```python
from build123d import *

# Parameters (mm, degrees)
BOSS_EXTRUDE1_DEPTH = 15
SKETCH6_R           = 15
SKETCH6_R_2         = 3
BOSS_EXTRUDE3_DEPTH = 15
CIRPATTERN3_COUNT   = 12


with BuildPart() as part:
    # Sketch1 → Boss-Extrude1 (new body, symmetric)
    with BuildSketch(Plane.XY):
        with BuildLine():
            Line((3, -13.07179677), (3, -9.801960973))
            ThreePointArc((3, -9.801960973), (-0.660686187, -16.827574978), (-0.232026419, -24.738082314))
            ThreePointArc((-0.232026419, -24.738082314), (0.803634844, -24.68419335), (1.8361294, -24.58696545))
            ThreePointArc((1.8361294, -24.58696545), (1.065897684, -18.692713773), (3, -13.07179677))
        make_face()
    boss_extrude1 = extrude(amount=BOSS_EXTRUDE1_DEPTH, both=True)

    # Sketch6 → Boss-Extrude3 (add, symmetric)
    with BuildSketch(Plane.XY):
        Circle(SKETCH6_R)
        Circle(SKETCH6_R_2, mode=Mode.SUBTRACT)
    extrude(amount=BOSS_EXTRUDE3_DEPTH, both=True)

    # CirPattern3: Boss-Extrude1 ×12 about axis
    cirpattern3_axis = Axis((0, 0, 0), (0, 0, 1))
    for i in range(1, CIRPATTERN3_COUNT):
        add(boss_extrude1.rotate(cirpattern3_axis, i * 360 / CIRPATTERN3_COUNT))


solid = part.part
```
Can you work these out from the model? Positions are in its coordinate system, mm. A direction names the side the tool comes from. Coordinates: 2 decimals unless noted, no trailing zeros. Loops run counter-clockwise (first coordinate to the right, second up) from the corner with the lowest first, then second, coordinate; pieces in that order, holes last.
1) I need wall thicknesses on probe 1 along Y at (x, z) = (0, 1.5); probe 2 along X at (y, z) = (-11, 7). Which ranges of each line are inside material? Lowest first, please.
2) Imagine slicing it at B-B on y = 16. List the corners of the cut face in (x, z) for me, plus the area to 3 significant figures.
3) Thinking about a two-plate mould opening in X: for faces 3 (the cylindrical face through (4.77, -14.22, 0.21)), 4 (the cylindrical face through (13, -21, 0)), 5 (the cylindrical face through (-24.685, -0.789, 0.21)), 6 (the flat face through (-5, -2, 15)), which applies, pulls with the +X half, pulls with the -X half, needs draft (parallel to the pull), parting line crosses it, or undercut?
4) For pin 1 (12 mm diameter, centred on x = 19.5, z = -10, fed in from -Y); pin 2 (8 mm diameter, centred on y = -15.5, z = 11, fed in from +X); pin 3 (12 mm diameter, centred on y = 15, z = -11.5, fed in from +X), each with a flat end and sliding along its axis, tell me the tip position at first contact or that it passes through.
5) Imagine slicing it at A-A on x = -18. List the corners of the cut face in (y, z) for me, plus the area to 3 significant figures.
6) Imagine slicing it at C-C on x = -6.5. List the corners of the cut face in (y, z) for me, plus the area to 3 significant figures.
7) Which directions (+Z, -Z, +X, -X, +Y, -Y) give clear straight access to the entire face, cutting with the end or side of a thin tool? Please do faces 1 (the cylindrical face through (-21, -13, 0)), 2 (the cylindrical face through (9.017, 17.623, 0.21)).
Completed:
1. probe 1: y = -24.73 to -3, 3 to 24.73
1. probe 2: x = -20.38 to -17.05, -10.2 to 10.2, 17.06 to 22.08
2. outline: (-10.43, -15) - (-8.24, -15) - (-8.24, 15) - (-10.43, 15) - close; (-1.63, -15) - (0.46, -15) - (0.46, 15) - (-1.63, 15) - close; (7.86, -15) - (10.36, -15) - (10.36, 15) - (7.86, 15) - close
2. area: 203 mm2
3. face 3: undercut
3. face 4: pulls with the +X half
3. face 5: pulls with the -X half
3. face 6: needs draft
4. pin 1: stops at y = -20.65
4. pin 2: stops at x = 21.85
4. pin 3: stops at x = 21.54
5. outline: (-11.64, -15) - (-9.24, -15) - (-9.24, 15) - (-11.64, 15) - close; (-1.15, -15) - (0.87, -15) - (0.87, 15) - (-1.15, 15) - close; (9.24, -15) - (11.48, -15) - (11.48, 15) - (9.24, 15) - close
5. area: 200 mm2
6. outline: (-14.59, -15) - (13.52, -15) - (13.52, 15) - (-14.59, 15) - close
6. area: 843 mm2
7. face 1: +Z, -Z, -X, -Y
7. face 2: +Z, -Z, +Y
